For this review, take the finished solid that the model builds, in its own axes (mm). A direction names the side the tool comes from. Give positions to 0.01 mm unless a question says otherwise; leave off trailing zeros. Loops run counter-clockwise (first coordinate to the right, second up) from the corner with the lowest first, then second, coordinate; pieces in that order, holes last.
```python
from build123d import *

# Parameters (mm, degrees)
PAD_DEPTH         = 77
SKETCH001_W       = 69
SKETCH001_H       = 52
PAD001_DEPTH      = 2
SKETCH002_R       = 1.5
POCKET_DEPTH      = 5.501
POCKET_DEPTH_BACK = -74.501
SKETCH003_W       = 2.5
SKETCH003_H       = 21
PAD002_DEPTH      = 3
SKETCH004_R       = 1.6
POCKET001_DEPTH   = 10
POCKET002_DEPTH   = 2.5


with BuildPart() as part:
    # Sketch → Pad (new body)
    with BuildSketch(Plane.XZ):
        Polygon((0, 0), (69, 0), (69, 50), (74.5, 50), (74.5, 52), (67, 52), (67, 2), (2, 2), (2, 52), (-5.5, 52), (-5.5, 50), (0, 50), align=None)
    extrude(amount=PAD_DEPTH)

    # Sketch001 → Pad001 (join)
    with BuildSketch(Plane.XZ):
        with Locations((34.5, 26)):
            Rectangle(SKETCH001_W, SKETCH001_H)
    extrude(amount=PAD001_DEPTH)

    # Sketch002 → Pocket (cut, two sides)
    with BuildSketch(Plane.YZ) as pocket_sk:
        with Locations((-75, 26)):
            Circle(SKETCH002_R)
    extrude(amount=-POCKET_DEPTH, mode=Mode.SUBTRACT)
    extrude(pocket_sk.sketch, amount=-POCKET_DEPTH_BACK, mode=Mode.SUBTRACT)

    # Sketch003 (on Face8 of Pocket) → Pad002 (join)
    with BuildSketch(Plane(origin=(0, 0, 52), x_dir=(-1, 0, 0), z_dir=(0, 0, 1))):
        with Locations((-68.25, 37.5)):
            Rectangle(SKETCH003_W, SKETCH003_H)
        with Locations((-0.75, 37.5)):
            Rectangle(SKETCH003_W, SKETCH003_H)
    extrude(amount=PAD002_DEPTH)

    # Sketch004 (on Face21 of Pad002) → Pocket001 (cut)
    with BuildSketch(Plane(origin=(0, 0, 55), x_dir=(-1, 0, 0), z_dir=(0, 0, 1))):
        with Locations((-68.25, 38)):
            Circle(SKETCH004_R)
        with Locations((-0.75, 38)):
            Circle(SKETCH004_R)
    extrude(amount=-POCKET001_DEPTH, mode=Mode.SUBTRACT)

    # Sketch005 (on Face11 of Pocket001) → Pocket002 (cut)
    with BuildSketch(Plane(origin=(0, 0, 50.5), x_dir=(-1, 0, 0), z_dir=(0, 0, 1))):
        Polygon((1.195, 34.631161), (3.14, 38), (1.195, 41.368839), (-2.695, 41.368839), (-4.64, 38), (-2.695, 34.631161), align=None)
        Polygon((-66.305, 34.631161), (-64.36, 38), (-66.305, 41.368839), (-70.195, 41.368839), (-72.14, 38), (-70.195, 34.631161), align=None)
    extrude(amount=-POCKET002_DEPTH, mode=Mode.SUBTRACT)


solid = part.part
```
Item 1: Take a section at A-A on z = 26. Give the boundary of the cut face in (x, y).
Answer:
outline: (0, -77) - (2, -77) - (2, -76.5) - (0, -76.5) - close; (0, -73.5) - (2, -73.5) - (2, -2) - (67, -2) - (67, -73.5) - (69, -73.5) - (69, 0) - (0, 0) - close; (67, -77) - (69, -77) - (69, -76.5) - (67, -76.5) - close
Item 2: Clearance check with flat-ended pins moving along their axes: pin 1 Ø1 at (x, z) = (5, 7) entering from -Y; pin 2 Ø0.8 at (x, z) = (0.5, 54) entering from +Y; pin 3 Ø3.5 at (y, z) = (-34, 54) entering from +X. State where each tip first meets the part, or that it passes through.
Answer:
pin 1: stops at y = -2
pin 2: stops at y = -27
pin 3: stops at x = 69.5
Item 3: Take a section at D-D on y = -31. Give the boundary of the cut face in (x, z), and give its area (3 significant figures).
Answer:
outline: (-5.5, 50) - (0, 50) - (0, 0) - (69, 0) - (69, 50) - (74.5, 50) - (74.5, 52) - (69.5, 52) - (69.5, 55) - (67, 55) - (67, 2) - (2, 2) - (2, 55) - (-0.5, 55) - (-0.5, 52) - (-5.5, 52) - close
area: 375 mm2
Item 4: Take a section at C-C on z = 13.5. Give the boundary of the cut face in (x, y), and give its area (3 significant figures).
Answer:
outline: (0, -77) - (2, -77) - (2, -2) - (67, -2) - (67, -77) - (69, -77) - (69, 0) - (0, 0) - close
area: 438 mm2
Item 5: Take a section at B-B on y = -75. Give the boundary of the cut face in (x, z), and give its area (3 significant figures).
Answer:
outline: (-5.5, 50) - (0, 50) - (0, 27.5) - (2, 27.5) - (2, 52) - (-5.5, 52) - close; (0, 0) - (69, 0) - (69, 24.5) - (67, 24.5) - (67, 2) - (2, 2) - (2, 24.5) - (0, 24.5) - close; (67, 27.5) - (69, 27.5) - (69, 50) - (74.5, 50) - (74.5, 52) - (67, 52) - close
area: 348 mm2
Item 6: The part is to be moulded in two halves that separate along X. For faces 1 (the cylindrical face through (1.09, -36.437, 46.521)), 2 (the flat face through (-5.5, -38, 51)), 3 (the flat face through (68, -48, 53)), 4 (the flat face through (74.5, -38, 51)), say which applies: released by +X, released by -X, zero draft, split by the parting line, or undercut.
Answer:
face 1: undercut
face 2: released by -X
face 3: zero draft
face 4: released by +X
Item 7: Tool access review of faces 5 (the flat face through (2, -39, 28)), 6 (the flat face through (69, -38, 25)), 7 (the cylindrical face through (67.91, -39.563, 46.521)), 8 (the flat face through (1, -41.369, 49)): name each direction out of +Z, -Z, +X, -X, +Y, -Y from which nothing blocks a thin tool from reaching the whole face with its end or side.
Answer:
face 5: +Z, -Y
face 6: -Z, +X, +Y, -Y
face 7: +Z
face 8: none
Item 8: For L1, parallel to Y at x = 0.6, z = 26; L2, parallel to X at y = -48.5, z = 10; L3, parallel to Y at x = 68.25, z = 52.35, list the stretches that pass through material, from the lowest coordinate up.
Answer:
L1: y = -77 to -76.5, -73.5 to 0
L2: x = 0 to 2, 67 to 69
L3: y = -48 to -39.6, -36.4 to -27
